Autodesk Inventor part; units mm, degrees
ref_plane "YZ Plane" through (0, 0, 0) normal (1, 0, 0) x (0, 1, 0)
ref_plane "XZ Plane" through (0, 0, 0) normal (0, 1, 0) x (-1, 0, 0)
ref_plane "XY Plane" through (0, 0, 0) normal (0, 0, 1) x (1, 0, 0)
sketch "Эскиз1" plane through (0, 0, 0) normal (0, 1, 0) x (-1, 0, 0)
  circle A0 centre (0, 0) radius 152.5
  line L0 (0, 0) -> (152.5, 0)
  circle A1 centre (87.5, 0) radius 65
  circle A2 centre (-43.75, 75.777223) radius 65
  circle A3 centre (-43.75, -75.777223) radius 65
  circle A4 centre (87.5, 0) radius 75
  circle A5 centre (-43.75, 75.777223) radius 75
  circle A6 centre (-43.75, -75.777223) radius 75
  line L1 (0, 0) -> (-76.25, 132.068874)
  line L2 (0, 0) -> (-76.25, -132.068874)
  line L3 (144.5, 48.74423) -> (30.5, -48.74423)
  line L4 (-114.463742, 100.768556) -> (26.963742, 50.78589)
  line L5 (-30.036258, -149.512786) -> (-57.463742, -2.04166)
  line L6 (30.5, -48.74423) -> (26.963742, -50.78589)
  line L7 (26.963742, 50.78589) -> (30.5, 48.74423)
  line L8 (-57.463742, -2.04166) -> (-57.463742, 2.04166)
  point P0 (14.069297, 24.368737)
  point P1 (-28.138593, 0)
  point P2 (14.069297, -24.368737)
  point P3 (12.5, 0)
  point P4 (22.5, 0)
  point P5 (152.5, 0)
  point P6 (-6.25, 10.825318)
  point P7 (-11.25, 19.485572)
  point P8 (-76.25, 132.068874)
  point P9 (-114.463742, 100.768556)
  point P10 (-6.25, -10.825318)
  point P11 (-11.25, -19.485572)
  point P12 (-76.25, -132.068874)
  point P13 (-30.036258, -149.512786)
  point P14 (-114.463742, -100.768556)
  point P15 (-30.036258, 149.512786)
  point P16 (144.5, -48.74423)
  point P17 (152.5, 0)
  point P18 (136.9, 42.245)
  point P19 (17.535243, 54.118068)
  point P20 (-105.035243, 97.436378)
  point P21 (-114.463742, 100.768556)
  point P22 (-57.463742, -2.04166)
  point P23 (-55.635243, -11.873068)
  point P24 (-31.864757, -139.681378)
  point P25 (-30.036258, -149.512786)
  point P26 (38.1, -42.245)
  dimension "d0" = 305
  dimension "d1" = 130
  dimension "d2" = 0
  dimension "d5" = 360
  dimension "d7" = 150
  dimension "d10" = 360
  dimension "d16" = 360
  dimension "d18" = 0
  dimension "d21" = 360
  dimension "d25" = 360
sketch "Эскиз1 outline for Выдавливание1" plane through (0, 0, 0) normal (0, 1, 0) x (-1, 0, 0)
  line L0 (136.9, 42.245) -> (144.5, 48.74423)
  arc A0 (38.1, -42.245) -> (136.9, 42.245) centre (87.5, 0) cw
  line L1 (30.5, -48.74423) -> (38.1, -42.245)
  line L2 (26.963742, -50.78589) -> (30.5, -48.74423)
  arc A1 (-30.036258, -149.512786) -> (26.963742, -50.78589) centre (-43.75, -75.777223) ccw
  line L3 (-31.864757, -139.681378) -> (-30.036258, -149.512786)
  arc A2 (-55.635243, -11.873068) -> (-31.864757, -139.681378) centre (-43.75, -75.777223) cw
  line L4 (-57.463742, -2.04166) -> (-55.635243, -11.873068)
  line L5 (-57.463742, 2.04166) -> (-57.463742, -2.04166)
  arc A3 (-114.463742, 100.768556) -> (-57.463742, 2.04166) centre (-43.75, 75.777223) ccw
  line L6 (-105.035243, 97.436378) -> (-114.463742, 100.768556)
  arc A4 (17.535243, 54.118068) -> (-105.035243, 97.436378) centre (-43.75, 75.777223) cw
  line L7 (26.963742, 50.78589) -> (17.535243, 54.118068)
  line L8 (30.5, 48.74423) -> (26.963742, 50.78589)
  arc A5 (144.5, 48.74423) -> (30.5, 48.74423) centre (87.5, 0) ccw
extrude "Выдавливание1" add sketch "Эскиз1 outline for Выдавливание1" along normal blind 10
chamfer "Фаска1" distance 10 angle 45 3 edges at (55.6352, 5, -11.8731) (-17.5352, 5, 54.1181) (-38.1, 5, -42.245)
sketch "Эскиз2" plane through (0, 10, 0) normal (0, 1, 0) x (1, 0, 0)
  line L0 (-32.204642, 34.167577) -> (-30.5, 48.74423)
  line L1 (-32.204642, 34.167577) -> (-31.020127, 86.842802)
  arc A0 (30.036258, 149.512786) -> (-26.963742, 50.78589) centre (43.75, 75.777223) ccw
  line L2 (-13.487669, -44.973827) -> (-59.698009, -70.285619)
  line L3 (45.692311, 10.806249) -> (90.718136, -16.557183)
  line L4 (-32.204642, 34.167577) -> (-30.5, 48.74423)
  arc A1 (-136.9, -42.245) -> (-32.204642, 34.167577) centre (-87.5, 0) ccw
  line L5 (-136.9, -42.245) -> (-144.5, -48.74423)
  arc A2 (-144.5, -48.74423) -> (-30.5, -48.74423) centre (-87.5, 0) ccw
  line L6 (-30.5, -48.74423) -> (-26.963742, -50.78589)
  line L7 (-13.487669, -44.973827) -> (-26.963742, -50.78589)
  arc A3 (105.035243, -97.436378) -> (-13.487669, -44.973827) centre (43.75, -75.777223) ccw
  line L8 (105.035243, -97.436378) -> (114.463742, -100.768556)
  arc A4 (114.463742, -100.768556) -> (57.463742, -2.04166) centre (43.75, -75.777223) ccw
  line L9 (57.463742, -2.04166) -> (57.463742, 2.04166)
  line L10 (45.692311, 10.806249) -> (57.463742, 2.04166)
  arc A5 (31.864757, 139.681378) -> (45.692311, 10.806249) centre (43.75, 75.777223) ccw
  line L11 (31.864757, 139.681378) -> (30.036258, 149.512786)
  arc A6 (30.036258, 149.512786) -> (-26.963742, 50.78589) centre (43.75, 75.777223) ccw
  line L12 (-26.963742, 50.78589) -> (-30.5, 48.74423)
  point P0 (0, 0)
  point P1 (82.700735, -11.684788)
  point P2 (-51.46969, -65.778544)
  point P3 (-31.231045, 77.463331)
  dimension "d32" = 360
sketch "Эскиз2 outline for Выдавливание2" plane through (0, 10, 0) normal (0, 1, 0) x (1, 0, 0)
  line L0 (57.463742, 2.04166) -> (57.463742, -2.04166)
  line L1 (45.692311, 10.806249) -> (57.463742, 2.04166)
  line L2 (82.700735, -11.684788) -> (45.692311, 10.806249)
  arc A0 (57.463742, -2.04166) -> (82.700735, -11.684788) centre (43.75, -75.777223) cw
  line L3 (-26.963742, -50.78589) -> (-30.5, -48.74423)
  line L4 (-13.487669, -44.973827) -> (-26.963742, -50.78589)
  line L5 (-51.46969, -65.778544) -> (-13.487669, -44.973827)
  arc A1 (-30.5, -48.74423) -> (-51.46969, -65.778544) centre (-87.5, 0) cw
  line L6 (-30.5, 48.74423) -> (-26.963742, 50.78589)
  line L7 (-32.204642, 34.167577) -> (-30.5, 48.74423)
  line L8 (-31.231045, 77.463331) -> (-32.204642, 34.167577)
  arc A2 (-26.963742, 50.78589) -> (-31.231045, 77.463331) centre (43.75, 75.777223) cw
extrude "Выдавливание2" add sketch "Эскиз2 outline for Выдавливание2" against normal blind 10
sketch "Эскиз3" plane through (0, 10, 0) normal (0, 1, 0) x (1, 0, 0)
  arc A0 (-136.9, -42.245) -> (-32.204642, 34.167577) centre (-87.5, 0) ccw
  line L0 (-136.9, -42.245) -> (-144.5, -48.74423)
  arc A1 (-144.5, -48.74423) -> (-51.46969, -65.778544) centre (-87.5, 0) ccw
  line L1 (-51.46969, -65.778544) -> (-13.487669, -44.973827)
  arc A2 (105.035243, -97.436378) -> (-13.487669, -44.973827) centre (43.75, -75.777223) ccw
  line L2 (105.035243, -97.436378) -> (114.463742, -100.768556)
  arc A3 (114.463742, -100.768556) -> (82.700735, -11.684788) centre (43.75, -75.777223) ccw
  line L3 (82.700735, -11.684788) -> (45.692311, 10.806249)
  arc A4 (31.864757, 139.681378) -> (45.692311, 10.806249) centre (43.75, 75.777223) ccw
  line L4 (31.864757, 139.681378) -> (30.036258, 149.512786)
  arc A5 (30.036258, 149.512786) -> (-31.231045, 77.463331) centre (43.75, 75.777223) ccw
  line L5 (-31.231045, 77.463331) -> (-32.204642, 34.167577)
  line L6 (-31.231045, 77.463331) -> (-15.37541, -56.235706)
  line L7 (-51.46969, -65.778544) -> (56.389255, 14.802358)
  line L8 (82.700735, -11.684788) -> (-41.013845, 41.433348)
  point P0 (0, 0)
  point P1 (4.846874, -23.704708)
  point P2 (18.105443, 16.04987)
  point P3 (-22.952316, 7.654838)
  dimension "d38" = 360
sketch "Эскиз3 outline for Выдавливание3" plane through (0, 10, 0) normal (0, 1, 0) x (1, 0, 0)
  line L0 (4.846874, -23.704708) -> (-51.46969, -65.778544)
  arc A0 (-13.487669, -44.973827) -> (4.846874, -23.704708) centre (43.75, -75.777223) cw
  line L1 (-51.46969, -65.778544) -> (-13.487669, -44.973827)
  line L2 (18.105443, 16.04987) -> (82.700735, -11.684788)
  arc A1 (45.692311, 10.806249) -> (18.105443, 16.04987) centre (43.75, 75.777223) cw
  line L3 (82.700735, -11.684788) -> (45.692311, 10.806249)
  line L4 (-22.952316, 7.654838) -> (-31.231045, 77.463331)
  arc A2 (-32.204642, 34.167577) -> (-22.952316, 7.654838) centre (-87.5, 0) cw
  line L5 (-31.231045, 77.463331) -> (-32.204642, 34.167577)
extrude "Выдавливание3" cut sketch "Эскиз3 outline for Выдавливание3" against normal through all
fillet "Сопряжение1" radius 20 3 edges at (82.7007, 5, 11.6848) (-51.4697, 5, 65.7785) (-31.231, 5, -77.4633)
sketch "Эскиз4" plane through (0, 10, 0) normal (0, 1, 0) x (1, 0, 0)
  circle A0 centre (0, 0) radius 4
  dimension "d43" = 8
sketch "Эскиз4 outline for Выдавливание4" plane through (0, 10, 0) normal (0, 1, 0) x (1, 0, 0)
  circle A0 centre (0, 0) radius 4
extrude "Выдавливание4" cut sketch "Эскиз4 outline for Выдавливание4" against normal blind 140
properties part number "сюрикен"
Build history of the part. All positions in model axes, mm. A direction names the side the tool comes from. Coordinates: 2 decimals unless noted, no trailing zeros. Order: outer loops, then holes, each group sorted by start corner. A loop starts at its lowest first (then second) coordinate and runs counter-clockwise, first axis right, second up. Notation, with made-up numbers: M 13.25,10 L 48.25,10 A6 ccw 48.25,21 Z; hole C 33,61.5 d6. An arc over 180 degrees is marked long. One line per question, with ' | ' between items. Start each with the question number.
Q1. Probe L1, parallel to Z at x = 0, y = 6.75; L2, parallel to X at y = 5.75, z = 0; L3, parallel to X at y = 3.5, z = 68. List the from-to ranges inside material, lowest first. Write a range as from..to.
Q2. 3-axis set-ups, long thin cutter, end or side, ignore diameter. For faces 5 (the face through (-26.946, 5.07, -41.328)), 6 (the face through (-13.27, 4.93, -124.5)), 7 (the face through (-60.366, 4.93, 59.066)): which of +Z, -Z, +X, -X, +Y, -Y reach the whole face in a straight line?
Q3. Two-plate mould, pull along X, no slides. Class faces 1 (the face through (109.68, 4.93, 99.08)), 2 (the face through (49.264, 5.07, -2.672)), 3 (the face through (-22.32, 5.07, 44)), 4 (the face through (-3, 0, 4)): +X half, -X half, draft (parallel to the pull), parting line (faces both ways), or undercut.
Q4. Saw through at C-C (z = 0). List the corners of the cut face in (x, y), then the cut area to 3 significant figures.
Q5. Flat gauge pins, fed straight in: pin 1 Ø1.5 at (x, y) = (22.5, 9) entering from +Z; pin 2 Ø1.5 at (y, z) = (3.5, -6.5) entering from -X; pin 3 Ø7 at (x, z) = (0, 0) entering from +Y; pin 4 Ø2 at (y, z) = (3.5, -63.5) entering from +X. Where does each tip first touch, or does it go through?
Q6. Saw through at D-D (z = -38). List the corners of the cut face in (x, y) (3 decimals).
Q7. Saw through at B-B (x = -26). List the corners of the cut face in (y, z).
Check values:
1) L1: z = -136.69..-123.85, -27.71..-4, 4..27.33 | L2: x = -22.5..-4, 4..55.49 | L3: x = -119.14..-55.86, 108.28..118.35
2) face 5: -X, +Y, -Y | face 6: -Z, -X, +Y, -Y | face 7: +Y, -Y
3) face 1: -X half | face 2: +X half | face 3: undercut | face 4: draft
4) outline: M -22.5,0 L -4,0 L -4,10 L -22.5,10 Z; M 4,0 L 55.49,0 L 55.49,10 L 4,10 Z | area: 700 mm2
5) pin 1: stops at z = 14.61 | pin 2: stops at x = -22.91 | pin 3: passes through | pin 4: stops at x = -19.88
6) outline: M -26.551,0 L -9.145,0 L -9.145,10 L -26.551,10 Z
7) outline: M 0,-103.34 L 10,-103.34 L 10,-33.35 L 0,-33.35 Z; M 0,21.04 L 10,21.04 L 10,46.75 L 0,46.75 Z
